Here's how the part is built. I have some questions about the finished solid (model axes, mm). A direction names the side the tool comes from. Coordinates: 2 decimals unless noted, no trailing zeros. Write each loop counter-clockwise with the first axis right and the second up, starting at its lowest first coordinate (ties: lowest second). Pieces come first, ordered by that corner, then holes.
(1) Thinking about a two-plate mould opening in X: for faces 1 (the cylindrical face through (-2.29, 13.78, -5.4)), 2 (the cylindrical face through (-5, 0, -10)), 3 (the flat face through (-7, 14, 0)), 4 (the cylindrical face through (-2.327, 13.776, 5.432)), which applies, released by +X, released by -X, zero draft, split by the parting line, or undercut?
(2) Imagine slicing it at C-C, the plane x = 7.5. List the corners of the cut face in (y, z) for me.
(3) Imagine slicing it at D-D, the plane y = 29.5. List the corners of the cut face in (x, z) for me, plus the area to 3 significant figures.
(4) Imagine slicing it at B-B, the plane y = 6.5. List the corners of the cut face in (x, z) for me.
(5) Which directions (+Z, -Z, +X, -X, +Y, -Y) give clear straight access to the entire face, cutting with the end or side of a thin tool? Please do faces 5 (the cylindrical face through (13.25, 0.03, 0.04)), 6 (the cylindrical face through (-5, 28, 10)), 7 (the flat face through (5, 0, 5)), 8 (the flat face through (5, 0, -5)).
(6) For pin 1 Ø3 at (x, y) = (6, -0.5) entering from -Z; pin 2 Ø1.2 at (x, y) = (6, 0) entering from +Z; pin 3 Ø4 at (x, z) = (7.5, -1) entering from +Y, each with a flat end and sliding along its axis, tell me the tip position at first contact or that it passes through.
(7) Imagine slicing it at A-A, the plane z = -10. List the corners of the cut face in (x, y) for me, plus the area to 3 significant figures.
(8) Please list where these lines run through material, in increasing order: probe 1 along Z at (x, y) = (-5.25, 3.5); probe 2 along Y at (x, z) = (-0.25, -4.25); probe 3 along Y at (x, z) = (10.75, -3).
Autodesk Inventor part; units mm, degrees
ref_plane "Work Plane1" through (-5, 0, 0) normal (1, 0, 0) x (0, 1, 0)
ref_plane "Work Plane2" through (-7, 0, 0) normal (1, 0, 0) x (0, 1, 0)
ref_plane "XZ Plane" through (0, 0, 0) normal (0, 1, 0) x (-1, 0, 0)
sketch "Sketch1" plane through (0, 0, 0) normal (0, 1, 0) x (-1, 0, 0)
  circle A0 centre (0, 0) radius 2.35
  circle A1 centre (0, 0) radius 5
  line L0 (0, 5) -> (-10, 5)
  arc A2 (-10, 5) -> (-10, -5) centre (-10, 0) ccw
  line L1 (-10, -5) -> (0, -5)
  line L2 (-8.5, 0) -> (-11.5, 0) construction
  line L3 (-8.5, 1.75) -> (-11.5, 1.75)
  line L4 (-11.5, -1.75) -> (-8.5, -1.75)
  arc A3 (-8.5, -1.75) -> (-8.5, 1.75) centre (-8.5, 0) ccw
  arc A4 (-11.5, 1.75) -> (-11.5, -1.75) centre (-11.5, 0) ccw
  dimension "d0" = 4.7
  dimension "d1" = 10
  dimension "d36" = 5
  dimension "d37" = 1.75
  dimension "d38" = 10
  dimension "d39" = 3
extrude "Extrusion1" add sketch "Sketch1" against normal blind 2 and the other way blind 2 contours A0 | A1 | A1 L1 A2 L0
extrude "Extrusion2" add sketch "Sketch1" along normal blind 30 contours A1
extrude "Extrusion3" add sketch "Sketch1" along normal blind 32 contours A0
ref_plane "Work Plane1" through (-5, 0, 0) normal (1, 0, 0) x (0, 1, 0)
ref_plane "Work Plane2" through (-7, 0, 0) normal (1, 0, 0) x (0, 1, 0)
sketch "Sketch2" plane through (-7, 0, 0) normal (1, 0, 0) x (0, 1, 0)
  line L0 (30, -15) -> (-2, -15)
  line L1 (-2, 15) -> (30, 15)
  line L2 (30, 15) -> (30, -15)
  line L3 (30, -5) -> (30, 5)
  line L4 (2, -5) -> (-2, -5)
  line L5 (-2, 5) -> (-2, -5)
  line L6 (2, 5) -> (-2, 5)
  line L7 (2, -5) -> (2, 5)
  line L8 (-2, -15) -> (-2, 15)
  point P0 (0, 0)
  dimension "d11" = 30
  dimension "d12" = 15
extrude "Extrusion4" add sketch "Sketch2" along normal blind 4
sketch "Sketch4" plane through (-7, 0, 0) normal (-1, 0, 0) x (0, 0, 1)
  line L0 (10, 26.5) -> (10, 1.5) construction
  line L1 (8.5, 26.5) -> (8.5, 1.5)
  line L2 (11.5, 1.5) -> (11.5, 26.5)
  arc A0 (11.5, 26.5) -> (8.5, 26.5) centre (10, 26.5) ccw
  arc A1 (8.5, 1.5) -> (11.5, 1.5) centre (10, 1.5) ccw
  line L3 (-10, 26.5) -> (-10, 1.5) construction
  line L4 (-11.5, 26.5) -> (-11.5, 1.5)
  line L5 (-8.5, 1.5) -> (-8.5, 26.5)
  arc A2 (-8.5, 26.5) -> (-11.5, 26.5) centre (-10, 26.5) ccw
  arc A3 (-11.5, 1.5) -> (-8.5, 1.5) centre (-10, 1.5) ccw
  line L6 (15, -2) -> (15, 30)
  line L7 (10, 14) -> (-10, 14) construction
  point P0 (0, 0)
  point P1 (15, 14)
  point P2 (0, 14)
  dimension "d30" = 20
  dimension "d31" = 1.5
  dimension "d32" = 25
extrude "Extrusion5" cut sketch "Sketch4" against normal up to surface (4 mm away)
fillet "Fillet1" radius 2 2 edges at (-3, 14, -4) (-3, 14, 4)
fillet "Fillet2" radius 4 4 edges at (-5, 30, 15) (-5, -2, 15) (-5, -2, -15) (-5, 30, -15)
properties part number "Pok Mk3 Yaw Motor Support" material "ABS Plastic"
Recorded:
1. face 1: undercut
1. face 2: zero draft
1. face 3: released by -X
1. face 4: undercut
2. outline: (-2, -5) - (2, -5) - (2, -1.44) - (-2, -1.44) - close; (-2, 1.44) - (2, 1.44) - (2, 5) - (-2, 5) - close
3. outline: (-7, -12.94) - (-3, -12.94) - (-3, -6.93) arc R2 cw to (-0.71, -4.95) arc R5 ccw (long way) to (-0.71, 4.95) arc R2 cw to (-3, 6.93) - (-3, 12.94) - (-7, 12.94) - close
3. area: 174 mm2
4. outline: (-7, -15) - (-3, -15) - (-3, -11.5) - (-7, -11.5) - close; (-7, -8.5) - (-3, -8.5) - (-3, -6.93) arc R2 cw to (-0.71, -4.95) arc R5 ccw (long way) to (-0.71, 4.95) arc R2 cw to (-3, 6.93) - (-3, 8.5) - (-7, 8.5) - close; (-7, 11.5) - (-3, 11.5) - (-3, 15) - (-7, 15) - close
5. face 5: +Y, -Y
5. face 6: +X, -X
5. face 7: +Z, +X, +Y, -Y
5. face 8: -Z, +X, +Y, -Y
6. pin 1: stops at z = -5
6. pin 2: stops at z = 5
6. pin 3: stops at y = 2
7. outline: (-7, -2) - (-3, -2) - (-3, 0) - (-7, 0) - close; (-7, 28) - (-3, 28) - (-3, 30) - (-7, 30) - close
7. area: 16.0 mm2
8. probe 1: z = -15 to -11.5, -8.5 to 8.5, 11.5 to 15
8. probe 2: y = -2 to 30
8. probe 3: y = -2 to 2
